For this review, take the finished solid that the model builds, in its own axes (mm). Give positions to 0.01 mm unless a question says otherwise; leave off trailing zeros. Order: outer loops, then holes, each group sorted by start corner. A loop starts at its lowest first (then second) coordinate and runs counter-clockwise, first axis right, second up. Notation, with made-up numbers: (71.25, 62.25) -> (118.25, 62.25) arc R24 cw to (118.25, 90.25) -> close; hole circle Ø6 at (54.5, 30.5). An arc over 180 degrees is marked (long way). Return JSON: item names as keys, results as strings. Group by question number.
1) Add section B-B (x = 49). Give the boundary of the cut face in (y, z), then the cut area to 3 significant figures.
2) Add section A-A (z = 15.5). Give the boundary of the cut face in (x, y).
3) Add section C-C (y = -25). Give the boundary of the cut face in (x, z), then the cut area to 3 significant figures.
4) The part is to be moulded in two halves that separate along Y. For faces 1 (the face through (29.75, -115.94, 38.29)), 2 (the face through (52, -125, 75.528)), 3 (the face through (33, -254, 30)), say which applies: released by +Y, released by -Y, zero draft, split by the parting line, or undercut.
5) To check wall thickness, follow line 1 along Z through (x, y) = (65, -240.5); line 2 along X through (y, z) = (-41.5, 34.5); line 3 along Z through (x, y) = (38, -89). State the ranges of each line that lie inside material, in increasing order.
from build123d import *

# Parameters (mm, degrees)
F0_W     = 85.677929
F0_H     = 75.528391
F1_DEPTH = 254
F2_R     = 18.645275
F3_DEPTH = 254.001
F5_DEPTH = 127


with BuildPart() as f1:
    # F0 (on Front) → F1 (new body)
    with BuildSketch(Plane.XZ):
        with Locations((42.838964, 37.764195)):
            Rectangle(F0_W, F0_H)
    extrude(amount=F1_DEPTH)

    # F2 (on face) → F3 (cut, through all)
    with BuildSketch(Plane.XZ.offset(254)):
        with Locations((48.073757, 45.977701)):
            Circle(F2_R)
    extrude(amount=-F3_DEPTH, mode=Mode.SUBTRACT)

    # F4 (on face) → F5 (cut)
    with BuildSketch(Plane.XY.offset(75.528391)):
        Polygon((64.327642, -98.35007), (26.675224, -87.756582), (32.912441, -144.928277), (56.481365, -161.33453), (45.67463, -126.652271), align=None)
    extrude(amount=-F5_DEPTH, mode=Mode.SUBTRACT)


solid = f1.part
Evaluation:
{
 "1": {"outline": "(-254, 0) -> (-156.13, 0) -> (-156.13, 27.36) -> (-254, 27.36) -> close; (-254, 64.6) -> (-156.13, 64.6) -> (-156.13, 75.53) -> (-254, 75.53) -> close; (-137.32, 0) -> (-121.61, 0) -> (-121.61, 27.36) -> (-137.32, 27.36) -> close; (-137.32, 64.6) -> (-121.61, 64.6) -> (-121.61, 75.53) -> (-137.32, 75.53) -> close; (-94.04, 0) -> (0, 0) -> (0, 27.36) -> (-94.04, 27.36) -> close; (-94.04, 64.6) -> (0, 64.6) -> (0, 75.53) -> (-94.04, 75.53) -> close", "area": "7,950 mm^2"},
 "2": {"outline": "(0, -254) -> (85.68, -254) -> (85.68, 0) -> (0, 0) -> close; hole (26.68, -87.76) -> (32.91, -144.93) -> (56.48, -161.33) -> (45.67, -126.65) -> (64.33, -98.35) -> close"},
 "3": {"outline": "(0, 0) -> (85.68, 0) -> (85.68, 75.53) -> (0, 75.53) -> close; hole circle Ø37.29 at (48.07, 45.98)", "area": "5,380 mm^2"},
 "4": {"face 1": "undercut", "face 2": "zero draft", "face 3": "released by -Y"},
 "5": {"line 1": "0 to 38.16, 53.8 to 75.53", "line 2": "0 to 33.38, 62.77 to 85.68", "line 3": "0 to 30.29, 61.67 to 75.53"}
}
